Here's the drawing with two shaded views (mm, measured from the low corner). I have some questions. Round coordinates to 2 decimals unless told otherwise and drop trailing zeros. Order: outer loops, then holes, each group sorted by start corner. A loop starts at its lowest first (then second) coordinate and runs counter-clockwise, first axis right, second up. Notation, with made-up numbers: (-2, 59) - (23, 59) arc R13 cw to (23, 63) - close; hole circle Ø9 at (-4, 80). An arc over 180 degrees is marked (long way). One line per item, written item: value.
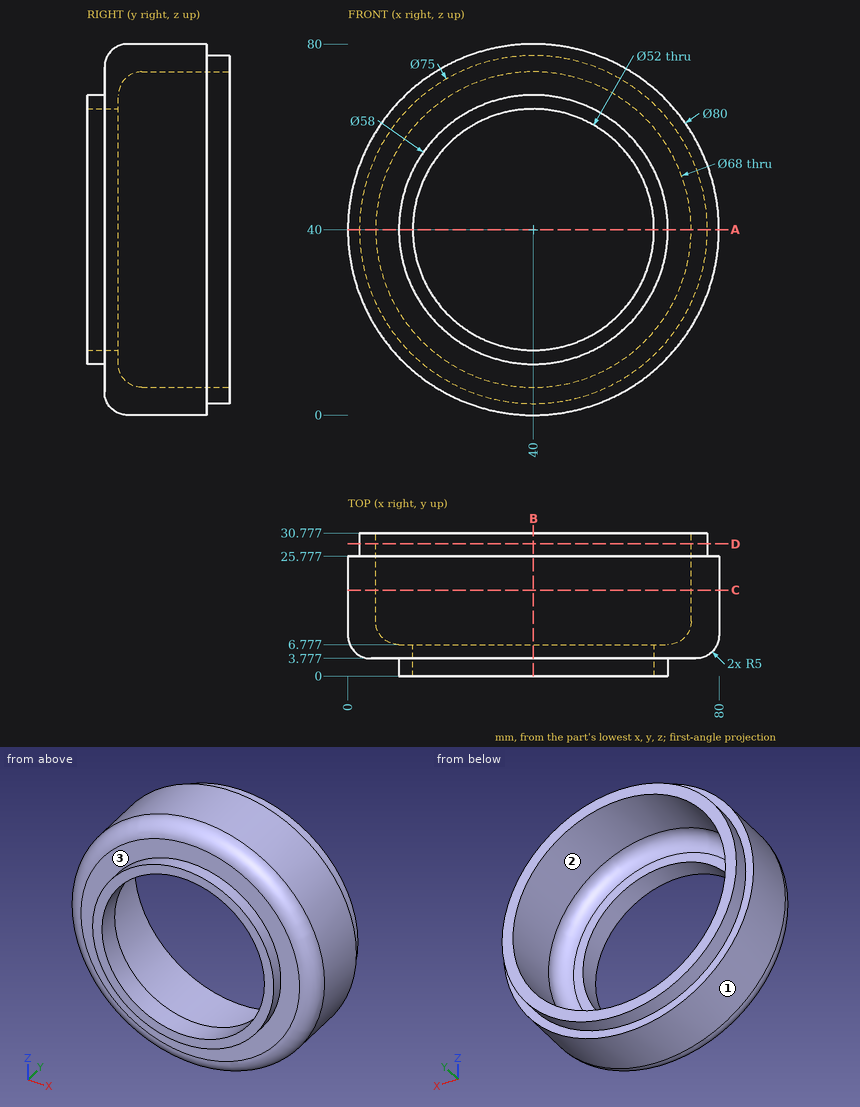
Q1. If we section it at D-D, the plane y = 28.5: Please give me the cut outline in (x, z), then the cut area to 3 significant figures.
Results list:
outline: circle Ø75 at (40, 40); hole circle Ø68 at (40, 40)
area: 786 mm²
Q2. If we section it at B-B, the plane x = 40: Please give me the cut outline in (y, z), then the cut area to 3 significant figures.
Results list:
outline: (0, 11) - (3.78, 11) - (3.78, 5) arc R5 ccw to (8.78, 0) - (25.78, 0) - (25.78, 2.5) - (30.78, 2.5) - (30.78, 6) - (11.78, 6) arc R5 cw to (6.78, 11) - (6.78, 14) - (0, 14) - close; (0, 66) - (6.78, 66) - (6.78, 69) arc R5 cw to (11.78, 74) - (30.78, 74) - (30.78, 77.5) - (25.78, 77.5) - (25.78, 80) - (8.78, 80) arc R5 ccw to (3.78, 75) - (3.78, 69) - (0, 69) - close
area: 370 mm²
Q3. Will these pins go through, and if not, where does the flat tip stop? pin 1 (12 mm diameter, centred on x = 41.5, y = 11.5, fed in from -Z); pin 2 (12 mm diameter, centred on x = 48, y = 20.5, fed in from +Z); pin 3 (2 mm diameter, centred on y = 7.5, z = 35, fed in from +X).
Results list:
pin 1: z = 0
pin 2: z = 79.95
pin 3: x = 79.74
Q4. If I drill on line 1 along Z through (x, y) = (40, 26); line 2 along Z through (x, y) = (40, 24), over which ranges is the centre line in solid material (lowest first)?
Results list:
line 1: 2.5 to 6, 74 to 77.5
line 2: 0 to 6, 74 to 80
Q5. If we section it at C-C, the plane y = 18.5: Please give me the cut outline in (x, z).
Results list:
outline: circle Ø80 at (40, 40); hole circle Ø68 at (40, 40)
Q6. We'd pull the mould along Z, two halves only. Please class the marked faces 1, 2 and 3: released by +Z, released by -Z, zero draft, split by the parting line, or undercut.
Results list:
face 1: split by the parting line
face 2: undercut
face 3: zero draft
Q7. If we section it at A-A, the plane z = 40: Please give me the cut outline in (x, y).
Results list:
outline: (0, 8.78) arc R5 ccw to (5, 3.78) - (11, 3.78) - (11, 0) - (14, 0) - (14, 6.78) - (11, 6.78) arc R5 cw to (6, 11.78) - (6, 30.78) - (2.5, 30.78) - (2.5, 25.78) - (0, 25.78) - close; (66, 0) - (69, 0) - (69, 3.78) - (75, 3.78) arc R5 ccw to (80, 8.78) - (80, 25.78) - (77.5, 25.78) - (77.5, 30.78) - (74, 30.78) - (74, 11.78) arc R5 cw to (69, 6.78) - (66, 6.78) - close
